Geometry check sheet. Reference: drawing and pictorial views, mm from the part's lowest x, y, z. Give positions to 0.01 mm unless a question says otherwise; leave off trailing zeros. Loops run counter-clockwise (first coordinate to the right, second up) from the corner with the lowest first, then second, coordinate; pieces in that order, holes last. Notation, with made-up numbers: (74.25, -34.75) -> (105.25, -34.75) arc R16 ccw to (105.25, -30.75) -> close; hole circle Ø6 at (-11.75, 48). An arc over 180 degrees is marked (long way). Answer in a Markdown table with one row per item. Add a question column.
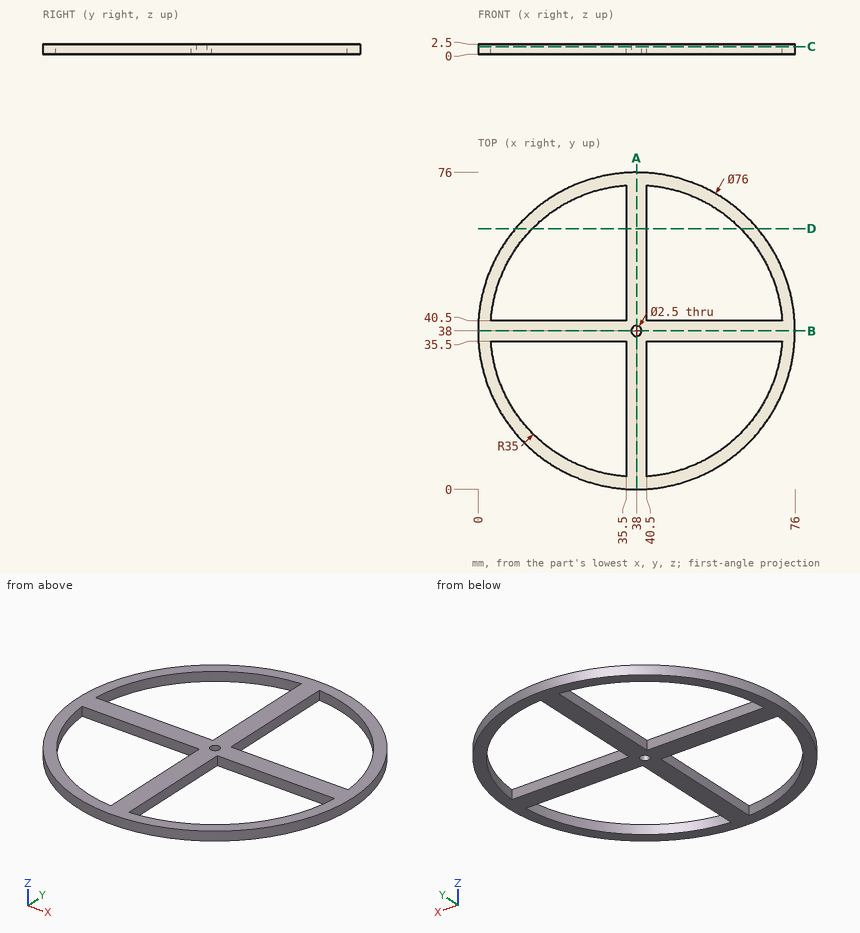
1. Gauge pin test, flat ends, axial feed: pin 1 Ø0.8 at (y, z) = (49.5, 2) entering from -X; pin 2 Ø1 at (y, z) = (48.5, 2) entering from -X; pin 3 Ø0.8 at (y, z) = (17.5, 0.5) entering from -X; pin 4 Ø10 at (x, y) = (29, 10) entering from -Z. Record the tip position at first contact, or that the pin passes through.
2. Material ranges on L1, parallel to X at y = 43.5, z = 0.15; L2, parallel to Y at x = 49, z = 1.85; L3, parallel to Y at x = 38, z = 0.9, recorded low to high. Write a range as from..to.
3. Sectioned sample at D-D (y = 62.5). Enter the section's corners in (x, z) (3 decimals).
4. Sectioned sample at C-C (z = 1.85). Enter the section's corners in (x, y).
5. Sectioned sample at A-A (x = 38). Enter the section's corners in (y, z), plus the area to 3 significant figures.
Response:
| question | item | result |
|---|---|---|
| 1 | pin 1 | stops at x = 1.66 |
| 1 | pin 2 | stops at x = 1.34 |
| 1 | pin 3 | stops at x = 5.75 |
| 1 | pin 4 | passes through |
| 2 | L1 | x = 0.4..3.43, 35.5..40.5, 72.57..75.6 |
| 2 | L2 | y = 1.63..4.77, 35.5..40.5, 71.23..74.37 |
| 2 | L3 | y = 0..36.75, 39.25..76 |
| 3 | outline | (8.953, 0) -> (13.005, 0) -> (13.005, 2.5) -> (8.953, 2.5) -> close; (35.5, 0) -> (40.5, 0) -> (40.5, 2.5) -> (35.5, 2.5) -> close; (62.995, 0) -> (67.047, 0) -> (67.047, 2.5) -> (62.995, 2.5) -> close |
| 4 | outline | circle Ø76 at (38, 38); hole (3.09, 35.5) arc R35 ccw to (35.5, 3.09) -> (35.5, 35.5) -> close; hole (3.09, 40.5) -> (35.5, 40.5) -> (35.5, 72.91) arc R35 ccw to start; hole circle Ø2.5 at (38, 38); hole (40.5, 3.09) arc R35 ccw to (72.91, 35.5) -> (40.5, 35.5) -> close; hole (40.5, 40.5) -> (72.91, 40.5) arc R35 ccw to (40.5, 72.91) -> close |
| 5 | outline | (0, 0) -> (36.75, 0) -> (36.75, 2.5) -> (0, 2.5) -> close; (39.25, 0) -> (76, 0) -> (76, 2.5) -> (39.25, 2.5) -> close |
| 5 | area | 184 mm2 |
